```python
from build123d import *

# Parameters (mm, degrees)
SKETCH1_W                    = 31.75
SKETCH1_H                    = 63.5
SKETCH1_W_2                  = 25.4
SKETCH1_H_2                  = 57.15
BOSS_EXTRUDE1_DEPTH          = 685.8
CUT_EXTRUDE1_REACH           = 691.238
F_10_0_1935_DIAMETER_HOLE1_D = 4.9149
CUT_EXTRUDE2_START           = -31.75
SKETCH6_R                    = 14.2875
SKETCH6_R_2                  = 3.2639
SKETCH6_R_3                  = 2.413
CUT_EXTRUDE2_DEPTH           = 31.75


with BuildPart() as part:
    # Sketch1 → Boss-Extrude1 (new body)
    with BuildSketch(Plane.XY):
        with Locations((3.710272719, -29.23968021)):
            Rectangle(SKETCH1_W, SKETCH1_H)
        with Locations((3.710272719, -29.23968021)):
            Rectangle(SKETCH1_W_2, SKETCH1_H_2, mode=Mode.SUBTRACT)
    extrude(amount=BOSS_EXTRUDE1_DEPTH)

    # Cut-Extrude1: up to this face of the body (flat: up to its plane)
    cut_extrude1_end = Plane(part.part.faces().sort_by_distance((19.585272719, -29.23968021, 342.9))[0])
    # Sketch3 → Cut-Extrude1 (cut, up to the picked face)
    with BuildSketch(Plane.ZY.offset(12.164727281), mode=Mode.PRIVATE) as cut_extrude1_sk1:
        with BuildLine():
            Line((31.7754, -13.36468021), (120.6754, -13.36468021))
            ThreePointArc((120.6754, -13.36468021), (122.92046403, -14.294616179), (123.8504, -16.53968021))
            Line((123.8504, -16.53968021), (123.8504, -41.93968021))
            ThreePointArc((123.8504, -41.93968021), (122.92046403, -44.18474424), (120.6754, -45.11468021))
            Line((120.6754, -45.11468021), (31.7754, -45.11468021))
            ThreePointArc((31.7754, -45.11468021), (29.53033597, -44.18474424), (28.6004, -41.93968021))
            Line((28.6004, -41.93968021), (28.6004, -16.53968021))
            ThreePointArc((28.6004, -16.53968021), (29.53033597, -14.294616179), (31.7754, -13.36468021))
        make_face()
    cut_extrude1_tool1 = split(extrude(cut_extrude1_sk1.sketch, amount=-CUT_EXTRUDE1_REACH, mode=Mode.PRIVATE), bisect_by=cut_extrude1_end, keep=Keep.BOTH, mode=Mode.PRIVATE)
    # Sketch3 → Cut-Extrude1 (cut, up to the picked face)
    with BuildSketch(Plane.ZY.offset(12.164727281), mode=Mode.PRIVATE) as cut_extrude1_sk2:
        with BuildLine():
            ThreePointArc((657.1996, -41.93968021), (656.26966403, -44.18474424), (654.0246, -45.11468021))
            Line((654.0246, -45.11468021), (565.1246, -45.11468021))
            ThreePointArc((565.1246, -45.11468021), (562.87953597, -44.18474424), (561.9496, -41.93968021))
            Line((561.9496, -41.93968021), (561.9496, -16.53968021))
            ThreePointArc((561.9496, -16.53968021), (562.87953597, -14.294616179), (565.1246, -13.36468021))
            Line((565.1246, -13.36468021), (654.0246, -13.36468021))
            ThreePointArc((654.0246, -13.36468021), (656.26966403, -14.294616179), (657.1996, -16.53968021))
            Line((657.1996, -16.53968021), (657.1996, -41.93968021))
        make_face()
    cut_extrude1_tool2 = split(extrude(cut_extrude1_sk2.sketch, amount=-CUT_EXTRUDE1_REACH, mode=Mode.PRIVATE), bisect_by=cut_extrude1_end, keep=Keep.BOTH, mode=Mode.PRIVATE)
    add(cut_extrude1_tool1.solids().sort_by(Axis((-12.164727, -29.23968, 76.2254), (1, 0, 0)))[0], mode=Mode.SUBTRACT)
    add(cut_extrude1_tool2.solids().sort_by(Axis((-12.164727, -29.23968, 609.5746), (1, 0, 0)))[0], mode=Mode.SUBTRACT)

    # #10 (0.1935) Diameter Hole1 (through all)
    with Locations(Plane(origin=(3.710272719, 2.51031979, 677.8625), x_dir=(1, 0, 0), z_dir=(0, 1, 0))):
        with Locations((0, 0), (0, 669.925)):
            Hole(F_10_0_1935_DIAMETER_HOLE1_D / 2)

    # Sketch6 → Cut-Extrude2 (cut)
    with BuildSketch(Plane(origin=(19.585272719, 0, 0), x_dir=(0, 0, -1), z_dir=(1, 0, 0)).offset(CUT_EXTRUDE2_START)):
        with Locations(Location((-342.9, -34.00218021, 0), (0, 0, 90))):
            Circle(SKETCH6_R)
        with Locations(Location((-383.54, -8.91968021, 0), (0, 0, 90))):
            Circle(SKETCH6_R_2)
        with Locations(Location((-251.46, -8.91968021, 0), (0, 0, 90))):
            Circle(SKETCH6_R_2)
        with Locations(Location((-317.5, -55.40168021, 0), (0, 0, 90))):
            Circle(SKETCH6_R_3)
    extrude(amount=CUT_EXTRUDE2_DEPTH, mode=Mode.SUBTRACT)


solid = part.part
```
Model file for the job. Use its own axes, mm. A direction names the side the tool comes from. Coordinates: 2 decimals unless noted, no trailing zeros. Loops run counter-clockwise (first coordinate to the right, second up) from the corner with the lowest first, then second, coordinate; pieces in that order, holes last. Notation, with made-up numbers: M 68,-30 L 90,-30 A11 cw 90,-9 Z; hole C -13.75,21.5 d4. An arc over 180 degrees is marked long. Use CSV: the item, a comma, the result in double quotes. Start each with the question number.
1. Two-plate mould, pull along Y, no slides. Class faces 1 (the flat face through (3, 2.51, 338)), 2 (the flat face through (4, -0.665, 338)), 3 (the flat face through (-12.165, -16, 338)), 4 (the flat face through (3, -60.99, 338)): pulls with the +Y half, pulls with the -Y half, needs draft (parallel to the pull), parting line crosses it, or undercut.
2. Band-saw the part on C-C, the plane y = -32. Give the number of separate pieces and of enclosed holes in the cut face, then the cut area to 3 significant figures.
3. Band-saw the part on A-A, the plane z = 605. List the corners of the cut face in (x, y).
4. Band-saw the part on D-D, the plane z = 342.9. List the corners of the cut face in (x, y), then the cut area to 3 significant figures.
5. Band-saw the part on B-B, the plane z = 504.5. List the corners of the cut face in (x, y).
6. Tool access for faces 5 (the flat face through (19.585, -16, 338)), 6 (the flat face through (16.41, -17, 338)): list every direction of +Z, -Z, +X, -X, +Y, -Y with a clear straight run to the whole face (end or side of a thin tool).
7. Probe probe 1 along X at (y, z) = (-52, 149); probe 2 along Y at (x, z) = (-4.5, 356.5); probe 3 along Y at (x, z) = (-11.05, 317.5). List the from-to ranges inside material, lowest first. Write a range as [from, to].
Entries:
1,face 1,"pulls with the +Y half"
1,face 2,"undercut"
1,face 3,"needs draft"
1,face 4,"pulls with the -Y half"
2,separate pieces,"8"
2,enclosed holes,"0"
2,area,"2,970 mm2"
3,outline,"M -12.16,-60.99 L 19.59,-60.99 L 19.59,-45.11 L 16.41,-45.11 L 16.41,-57.81 L -8.99,-57.81 L -8.99,-45.11 L -12.16,-45.11 Z; M -12.16,-13.36 L -8.99,-13.36 L -8.99,-0.66 L 16.41,-0.66 L 16.41,-13.36 L 19.59,-13.36 L 19.59,2.51 L -12.16,2.51 Z"
4,outline,"M -12.16,-60.99 L 19.59,-60.99 L 19.59,-48.29 L 16.41,-48.29 L 16.41,-57.81 L -8.99,-57.81 L -8.99,-48.29 L -12.16,-48.29 Z; M -12.16,-19.71 L -8.99,-19.71 L -8.99,-0.66 L 16.41,-0.66 L 16.41,-19.71 L 19.59,-19.71 L 19.59,2.51 L -12.16,2.51 Z"
4,area,"383 mm2"
5,outline,"M -12.16,-60.99 L 19.59,-60.99 L 19.59,2.51 L -12.16,2.51 Z; hole M -8.99,-57.81 L 16.41,-57.81 L 16.41,-0.66 L -8.99,-0.66 Z"
6,face 5,"+Z, -Z, +X, +Y, -Y"
6,face 6,"+Z, -Z"
7,probe 1,"x = [-12.16, -8.99], [16.41, 19.59]"
7,probe 2,"y = [-60.99, -57.81], [-0.66, 2.51]"
7,probe 3,"y = [-60.99, -57.81], [-52.99, 2.51]"
